The listing builds one solid part. Answer for the finished solid, in the listing's coordinates (mm). Face numbers are marked on the shaded views. A direction names the side the tool comes from. Coordinates: 2 decimals unless noted, no trailing zeros. Loops run counter-clockwise (first coordinate to the right, second up) from the corner with the lowest first, then second, coordinate; pieces in that order, holes last. Notation, with made-up numbers: M 24.25,29 L 35.25,29 A23 ccw 35.25,37 Z; hole C 1,34.25 d11. An arc over 180 degrees is marked long. Answer as a JSON object with one key per item and string values. Group by question number.
1. For the marked faces 1, 2 and 3, determine the directions among +Z, -Z, +X, -X, +Y, -Y from which every point of the face is accessible in a straight line to the end or side of a thin tool.
2. A cutting plane is placed at C-C on z = -4.25. Give the vertices of the cut face in (x, y).
3. A cutting plane is placed at A-A on z = -2.75. Give the vertices of the cut face in (x, y).
4. A cutting plane is placed at B-B on y = -8.8. Give the vertices of the cut face in (x, z), and give its area (3 significant figures).
5. Given pin 1 (0.8 mm diameter, centred on x = 3.5, y = -5.5, fed in from +Z); pin 2 (1.8 mm diameter, centred on y = -8.8, z = -4.25, fed in from -X); pin 3 (1 mm diameter, centred on x = -0.5, z = -1, fed in from -Y); pin 4 (1.5 mm diameter, centred on x = 2, y = -3.5, fed in from +Z), each flat-ended and moving along its own axis, determine where each tip first touches the part or whether it passes through.
6. Straight lines are drawn through the part: L1, parallel to Y at x = -3.55, z = -4.25; L2, parallel to Z at x = -3.7, y = -8.8; L3, parallel to X at y = 5.75, z = -6. For each, find the intervals that lie inside material, in ascending order.
7. Determine the mould class of the marked faces 4, 5 and 6 for opening direction Z: released by +Z, released by -Z, zero draft, split by the parting line, or undercut.
8. A cutting plane is placed at D-D on y = -1.75. Give the vertices of the cut face in (x, z).
from build123d import *

# Parameters (mm, degrees)
CROQUIS1_W                         = 8
CROQUIS1_H                         = 21
BRIDA_BASE1_DEPTH                  = 1
BRIDA_DE_ARISTA1_STRIP_W           = 5.4732
BRIDA_DE_ARISTA1_STRIP_H           = 1
BRIDA_DE_ARISTA1_STRIP_CUT_DEPTH   = 21
BRIDA_DE_ARISTA1_STRIP_2_W         = 5.4732
BRIDA_DE_ARISTA1_STRIP_2_H         = 1
BRIDA_DE_ARISTA1_STRIP_CUT_2_DEPTH = 21
BRIDA_DE_ARISTA1_DEPTH             = 21
BRIDA_DE_ARISTA1_BEND_DEPTH        = 21
CROQUIS34_W                        = 2
CROQUIS34_H                        = 7
CORTAR_EXTRUIR1_DEPTH              = 10
CORTAR_EXTRUIR2_REACH              = 16.714
CROQUIS35_R                        = 1


# Sheet-metal steps are written as plain solids
with BuildPart() as part:
    # Croquis1 → Brida base1 (new body)
    with BuildSketch(Plane.XY):
        Rectangle(CROQUIS1_W, CROQUIS1_H)
    extrude(amount=-BRIDA_BASE1_DEPTH)

    # Brida de arista1 strip (across the edge) → Brida de arista1 strip cut (cut)
    with BuildSketch(Plane(origin=(-4, -10.5, -1), x_dir=(1, 0, 0), z_dir=(0, 1, 0))):
        with Locations((-1, -0.5)):
            Rectangle(BRIDA_DE_ARISTA1_STRIP_W, BRIDA_DE_ARISTA1_STRIP_H)
    extrude(amount=BRIDA_DE_ARISTA1_STRIP_CUT_DEPTH, mode=Mode.SUBTRACT)

    # Brida de arista1 strip 2 (across the edge) → Brida de arista1 strip cut 2 (cut)
    with BuildSketch(Plane(origin=(4, 10.5, -1), x_dir=(-1, 0, 0), z_dir=(0, -1, 0))):
        with Locations((-1, -0.5)):
            Rectangle(BRIDA_DE_ARISTA1_STRIP_2_W, BRIDA_DE_ARISTA1_STRIP_2_H)
    extrude(amount=BRIDA_DE_ARISTA1_STRIP_CUT_2_DEPTH, mode=Mode.SUBTRACT)

    # Brida de arista1 section (across the edge) → Brida de arista1 (add)
    with BuildSketch(Plane(origin=(-4, -10.5, -1), x_dir=(1, 0, 0), z_dir=(0, 1, 0))):
        with BuildLine():
            Line((0, 0.7366), (0, 5.5))
            Line((0, 5.5), (1, 5.5))
            Line((1, 5.5), (1, 0.7366))
            ThreePointArc((1, 0.7366), (1.215745145, 0.215745145), (1.7366, 0))
            Line((1.7366, 0), (1.7366, -1))
            ThreePointArc((1.7366, -1), (0.508638364, -0.491361636), (0, 0.7366))
        make_face()
    extrude(amount=BRIDA_DE_ARISTA1_DEPTH)

    # Brida de arista1 section 2 (across the edge) → Brida de arista1 bend (add)
    with BuildSketch(Plane(origin=(4, 10.5, -1), x_dir=(-1, 0, 0), z_dir=(0, -1, 0))):
        with BuildLine():
            Line((0, 0.7366), (0, 5.5))
            Line((0, 5.5), (1, 5.5))
            Line((1, 5.5), (1, 0.7366))
            ThreePointArc((1, 0.7366), (1.215745145, 0.215745145), (1.7366, 0))
            Line((1.7366, 0), (1.7366, -1))
            ThreePointArc((1.7366, -1), (0.508638364, -0.491361636), (0, 0.7366))
        make_face()
    extrude(amount=BRIDA_DE_ARISTA1_BEND_DEPTH)

    # Croquis34 → Cortar-Extruir1 (cut)
    with BuildSketch(Plane(origin=(4, 0, 0), x_dir=(0, 0, -1), z_dir=(1, 0, 0))):
        with Locations((1, 7)):
            Rectangle(CROQUIS34_W, CROQUIS34_H)
        with Locations((1, -7)):
            Rectangle(CROQUIS34_W, CROQUIS34_H)
    extrude(amount=-CORTAR_EXTRUIR1_DEPTH, mode=Mode.SUBTRACT)

    # Cortar-Extruir2: up to this face of the body (flat: up to its plane)
    cortar_extruir2_end = Plane(part.part.faces().sort_by_distance((-4, 0, -4.204419709))[0])
    # Croquis35 → Cortar-Extruir2 (cut, up to the picked face)
    with BuildSketch(Plane(origin=(4, 0, 0), x_dir=(0, 0, -1), z_dir=(1, 0, 0)), mode=Mode.PRIVATE) as cortar_extruir2_sk1:
        with Locations((4.25, 8.8)):
            Circle(CROQUIS35_R)
    cortar_extruir2_tool1 = split(extrude(cortar_extruir2_sk1.sketch, amount=-CORTAR_EXTRUIR2_REACH, mode=Mode.PRIVATE), bisect_by=cortar_extruir2_end, keep=Keep.BOTH, mode=Mode.PRIVATE)
    # Croquis35 → Cortar-Extruir2 (cut, up to the picked face)
    with BuildSketch(Plane(origin=(4, 0, 0), x_dir=(0, 0, -1), z_dir=(1, 0, 0)), mode=Mode.PRIVATE) as cortar_extruir2_sk2:
        with Locations(Location((4.25, -8.8, 0), (0, 0, 180))):
            Circle(CROQUIS35_R)
    cortar_extruir2_tool2 = split(extrude(cortar_extruir2_sk2.sketch, amount=-CORTAR_EXTRUIR2_REACH, mode=Mode.PRIVATE), bisect_by=cortar_extruir2_end, keep=Keep.BOTH, mode=Mode.PRIVATE)
    add(cortar_extruir2_tool1.solids().sort_by(Axis((4, 8.8, -4.25), (-1, 0, 0)))[0], mode=Mode.SUBTRACT)
    add(cortar_extruir2_tool2.solids().sort_by(Axis((4, -8.8, -4.25), (-1, 0, 0)))[0], mode=Mode.SUBTRACT)


solid = part.part
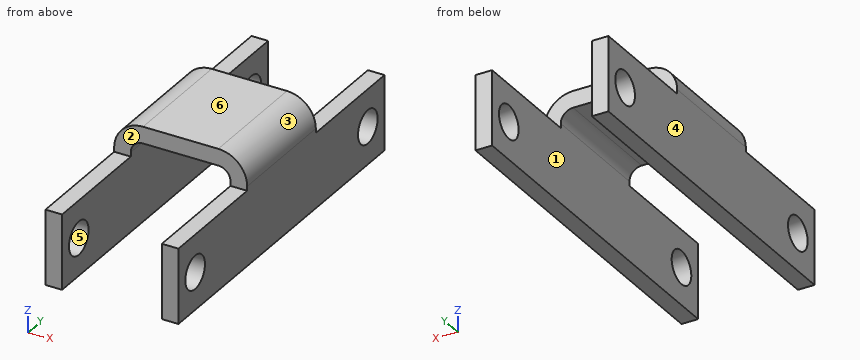
From the geometry:
{
 "1": {"face 1": "-Z, +Y, -Y", "face 2": "+Z, +X, -X, -Y", "face 3": "+Z, +X, +Y, -Y"},
 "2": {"outline": "M -4,-10.5 L -3,-10.5 L -3,-9.8 L -4,-9.8 Z; M -4,-7.8 L -3,-7.8 L -3,7.8 L -4,7.8 Z; M -4,9.8 L -3,9.8 L -3,10.5 L -4,10.5 Z; M 3,-10.5 L 4,-10.5 L 4,-9.8 L 3,-9.8 Z; M 3,-7.8 L 4,-7.8 L 4,7.8 L 3,7.8 Z; M 3,9.8 L 4,9.8 L 4,10.5 L 3,10.5 Z"},
 "3": {"outline": "M -4,-10.5 L -3,-10.5 L -3,10.5 L -4,10.5 Z; M 3,-10.5 L 4,-10.5 L 4,10.5 L 3,10.5 Z"},
 "4": {"outline": "M -4,-6.5 L -3,-6.5 L -3,-5.25 L -4,-5.25 Z; M -4,-3.25 L -3,-3.25 L -3,-2 L -4,-2 Z; M 3,-6.5 L 4,-6.5 L 4,-5.25 L 3,-5.25 Z; M 3,-3.25 L 4,-3.25 L 4,-2 L 3,-2 Z", "area": "5.00 mm²"},
 "5": {"pin 1": "stops at z = -2", "pin 2": "passes through", "pin 3": "stops at y = -3.5", "pin 4": "stops at z = 0"},
 "6": {"L1": "y = -10.5 to -9.8, -7.8 to 7.8, 9.8 to 10.5", "L2": "z = -6.5 to -5.25, -3.25 to -2", "L3": "x = -4 to -3, 3 to 4"},
 "7": {"face 4": "zero draft", "face 5": "undercut", "face 6": "released by +Z"},
 "8": {"outline": "M -4,-6.5 L -3,-6.5 L -3,-1.74 A0.74 cw -2.26,-1 L 2.26,-1 A0.74 cw 3,-1.74 L 3,-6.5 L 4,-6.5 L 4,-1.74 A1.74 ccw 2.26,0 L -2.26,0 A1.74 ccw -4,-1.74 Z"}
}
